Autodesk Fusion 360 part; units mm, degrees
sketch "Esquisse1" plane through (0, 0, 0) normal (0, 0, 1) x (1, 0, 0)
  line L0 (0, 0) -> (51, 0) construction
  line L1 (51, 0) -> (51, 36.5) construction
  line L2 (51, 36.5) -> (0, 36.5) construction
  line L3 (0, 36.5) -> (0, 0) construction
  circle A0 centre (0, 36.5) radius 1.2
  circle A1 centre (51, 36.5) radius 1.2
  circle A2 centre (0, 0) radius 1.2
  circle A3 centre (51, 0) radius 1.2
  line L4 (0, 18.25) -> (51, 18.25) construction
  line L5 (25.5, 36.5) -> (25.5, 0) construction
  line L6 (55.28, 41.85) -> (-4.28, 41.85)
  line L7 (-6.5, 39.63) -> (-6.5, -3.13)
  line L8 (-4.28, -5.35) -> (55.28, -5.35)
  line L9 (57.5, -3.13) -> (57.5, 39.63)
  line L10 (57.5, 41.85) -> (-6.5, -5.35) construction
  line L11 (-6.5, 41.85) -> (57.5, -5.35) construction
  line L12 (50.325, 36.86) -> (0.675, -0.36) construction
  line L13 (0.675, 36.86) -> (50.325, -0.36) construction
  line L14 (-5.3, 39.65) -> (-5.3, -3.15)
  line L15 (-4.3, -4.15) -> (55.3, -4.15)
  line L16 (56.3, -3.15) -> (56.3, 39.65)
  line L17 (55.3, 40.65) -> (-4.3, 40.65)
  arc A4 (-4.3, 40.65) -> (-5.3, 39.65) centre (-4.3, 39.65) ccw
  arc A5 (56.3, 39.65) -> (55.3, 40.65) centre (55.3, 39.65) ccw
  arc A6 (55.3, -4.15) -> (56.3, -3.15) centre (55.3, -3.15) ccw
  arc A7 (-5.3, -3.15) -> (-4.3, -4.15) centre (-4.3, -3.15) ccw
  arc A8 (57.5, 39.63) -> (55.28, 41.85) centre (55.28, 39.63) ccw
  arc A9 (-4.28, 41.85) -> (-6.5, 39.63) centre (-4.28, 39.63) ccw
  arc A10 (-6.5, -3.13) -> (-4.28, -5.35) centre (-4.28, -3.13) ccw
  arc A11 (55.28, -5.35) -> (57.5, -3.13) centre (55.28, -3.13) ccw
  line L18 (3, 37.05) -> (48, 37.05)
  line L19 (48, 37.05) -> (48, 30.05)
  line L20 (48, 30.05) -> (3, 30.05)
  line L21 (3, 30.05) -> (3, 37.05)
  line L22 (2, 38.05) -> (49, 38.05)
  line L23 (49, 38.05) -> (49, 29.05)
  line L24 (49, 29.05) -> (2, 29.05)
  line L25 (2, 29.05) -> (2, 38.05)
  line L26 (12.5, -4.15) -> (12.5, -5.35)
  line L27 (38.5, -4.15) -> (38.5, -5.35)
  line L28 (57.5, -3.13) -> (57.5, -13.13)
  line L29 (55.28, -15.35) -> (-4.28, -15.35)
  line L30 (-6.5, -13.13) -> (-6.5, -3.13)
  line L31 (56.3, -3.13) -> (56.3, -13.15)
  line L32 (55.3, -14.15) -> (-4.3, -14.15)
  line L33 (-5.3, -13.15) -> (-5.3, -3.13)
  arc A12 (-5.3, -13.15) -> (-4.3, -14.15) centre (-4.3, -13.15) ccw
  arc A13 (55.3, -14.15) -> (56.3, -13.15) centre (55.3, -13.15) ccw
  arc A14 (55.28, -15.35) -> (57.5, -13.13) centre (55.28, -13.13) ccw
  arc A15 (-6.5, -13.13) -> (-4.28, -15.35) centre (-4.28, -13.13) ccw
  point P0 (25.5, 18.25)
  point P1 (25.5, 18.25)
  dimension "d1" = 51
  dimension "d2" = 36.5
  dimension "d3" = 2.4
  dimension "d4" = 2.4
  dimension "d5" = 2.4
  dimension "d6" = 2.4
  dimension "d7" = 64
  dimension "d8" = 47.2
  dimension "d9" = 49.65
  dimension "d10" = 37.22
  dimension "d16" = 1
  dimension "d17" = 2.22
  dimension "d21" = 9.5
  dimension "d22" = 9.5
  dimension "d23" = 4.8
  dimension "d24" = 11.8
  dimension "d25" = -1
  dimension "d28" = 13
  dimension "d29" = 10
  dimension "d31" = 1
  dimension "d32" = 2.22
extrude "Extrusion1" add sketch "Esquisse1" along normal blind 1 contours L8 A10 A11 L31 L32 L33 A12 A13 | L8 L15 A6 A11 L27 L31 | L8 L15 A7 A10 L26 L33 | L14 L15 L16 L17 A4 A5 A6 A7 L31 L33 | L8 L15 L26 L27 | L22 L23 L24 L25
extrude "Extrusion2" add sketch "Esquisse1" along normal blind 11.8 contours L6 L7 L9 L14 L16 L17 A4 A5 A8 A9 A10 A11 L31 L33 | L8 L15 A6 A11 L27 L31 | L8 L15 A7 A10 L26 L33
chamfer "Chanfrein1" distance 1 angle 45 4 edges at (-1.1188, 0.4339, 0) (49.8812, 0.4339, 0) (49.8812, 36.9339, 0) (-1.1188, 36.9339, 0)
extrude "Extrusion3" add sketch "Esquisse1" along normal blind 4 contours L8 L15 L26 L27 | L22 L23 L24 L25
extrude "Extrusion4" add sketch "Esquisse1" along normal blind 10 contours A10 A11 L28 L29 L30 L31 L32 L33 A12 A13 A14 A15
equation "d4 = d3"
equation "d5 = d3"
equation "d6 = d3"
Part model, mm, in its own coordinate system. A direction names the side the tool comes from. Coordinates: 2 decimals unless noted, no trailing zeros. Write each loop counter-clockwise with the first axis right and the second up, starting at its lowest first coordinate (ties: lowest second). Pieces come first, ordered by that corner, then holes.
Item 1: Pin check, flat tips, straight feed: pin 1 (1 mm diameter, centred on x = 30.5, y = -5, fed in from +Z); pin 2 (3 mm diameter, centred on x = 0, y = 0, fed in from -Z); pin 3 (4.5 mm diameter, centred on x = 33, y = -8.5, fed in from +Z). Stop position of each tip, or through.
Item 2: Slice it at A-A (z = 3). Count the separate pieces of the cut face and the enclosed holes in it, and give its area (3 significant figures).
Item 3: Slice it at B-B (x = 18.5). Write the cut outline in (y, z).
Item 4: Which spindle directions (+Z, -Z, +X, -X, +Y, -Y) get a long thin tool onto all of the face, cutting with end or side? Do faces 4 (the face through (26, -14.15, 5)), 5 (the face through (57.5, 14, 6)), 6 (the face through (26, 30.05, 2)). Say none if no direction does.
Item 5: Probe line 1 (Y direction, x = 46.5, z = 7.5); line 2 (Y direction, x = 13, z = 1.75); line 3 (X direction, y = -3, z = 5.75). List the from-to ranges inside material, lowest first.
Item 6: Mould opens along X. For faces 1 (the face through (25, -5.35, 3)), 2 (the face through (25, 14, 0)), 3 (the face through (-5.83, -14.72, 4.93)) say: released by +X, released by -X, zero draft, split by the parting line, or undercut.
Results found:
1. pin 1: stops at z = 4
1. pin 2: stops at z = 0.7
1. pin 3: stops at z = 1
2. separate pieces: 2
2. enclosed holes: 3
2. area: 464 mm2
3. outline: (-15.35, 0) - (30.05, 0) - (30.05, 4) - (29.05, 4) - (29.05, 1) - (-4.15, 1) - (-4.15, 4) - (-5.35, 4) - (-5.35, 1) - (-14.15, 1) - (-14.15, 10) - (-15.35, 10) - close; (37.05, 0) - (41.85, 0) - (41.85, 11.8) - (40.65, 11.8) - (40.65, 1) - (38.05, 1) - (38.05, 4) - (37.05, 4) - close
4. face 4: +Z
4. face 5: +Z, -Z, +X, +Y, -Y
4. face 6: +Z, -Z
5. line 1: y = -15.35 to -14.15, -5.35 to -4.15, 40.65 to 41.85
5. line 2: y = -15.35 to -14.15, -5.35 to -4.15, 29.05 to 30.05, 37.05 to 38.05, 40.65 to 41.85
5. line 3: x = -6.5 to -5.3, 56.3 to 57.5
6. face 1: undercut
6. face 2: zero draft
6. face 3: released by -X
